```python
from build123d import *

# Parameters (mm, degrees)
SKETCH_1_W          = 60
SKETCH_1_H          = 45
EXTRUDE_1_DEPTH     = 13.5
CHAMFER_1_SIZE      = 10
FILLET_1_R          = 5
SHELL_1_T           = -1.5
FILLET_2_R          = 0.1
SKETCH_4_W          = 42
SKETCH_4_H          = 24
SKETCH_4_W_2        = 38
SKETCH_4_H_2        = 20
EXTRUDE_1_2_DEPTH   = 1
CUT_EXTRUDE_1_REACH = 47.349
SKETCH_7_R          = 2.5


with BuildPart() as part:
    # 草图1 → Extrude 1 (new, symmetric)
    with BuildSketch(Plane(origin=(0, 0, 0), x_dir=(1, 0, 0), z_dir=(0, 1, 0))):
        Rectangle(SKETCH_1_W, SKETCH_1_H)
    extrude(amount=EXTRUDE_1_DEPTH, both=True)

    # 倒角1
    chamfer_1_edges = [part.edges().sort_by_distance(p)[0] for p in [
        (-30, 0, 22.5),
        (-30, 0, -22.5),
    ]]
    chamfer(chamfer_1_edges, length=CHAMFER_1_SIZE)

    # 圆角1
    fillet_1_edges = [part.edges().sort_by_distance(p)[0] for p in [
        (-30, 0, 12.5),
        (-30, 0, -12.5),
        (-20, 0, -22.5),
        (-20, 0, 22.5),
    ]]
    fillet(fillet_1_edges, radius=FILLET_1_R)

    # 抽壳1
    shell_1_openings = [part.faces().sort_by_distance(p)[0] for p in [
        (30, 0, 0),
    ]]
    offset(amount=SHELL_1_T, openings=shell_1_openings, kind=Kind.INTERSECTION)

    # 圆角2
    fillet_2_edges = [part.edges().sort_by_distance(p)[0] for p in [
        (-25, 13.5, -17.5),
        (-30, 13.5, 0),
        (-25, 13.5, 17.5),
        (6.035533906, 13.5, 22.5),
        (-19.84234935, 13.5, 22.119397663),
        (-29.619397663, 13.5, 12.34234935),
        (-29.619397663, 13.5, -12.34234935),
        (-19.84234935, 13.5, -22.119397663),
        (-25, -13.5, -17.5),
        (-30, -13.5, 0),
        (6.035533906, -13.5, 22.5),
        (-25, -13.5, 17.5),
        (-19.84234935, -13.5, 22.119397663),
        (-29.619397663, -13.5, 12.34234935),
        (-29.619397663, -13.5, -12.34234935),
        (-19.84234935, -13.5, -22.119397663),
        (30, 13.5, 0),
        (6.035533906, -13.5, -22.5),
        (30, -12, 0),
        (30, 0, 21),
        (30, 0, -21),
        (30, 12, 0),
        (30, -13.5, 0),
        (6.035533906, 13.5, -22.5),
        (30, 0, 22.5),
        (30, 0, -22.5),
    ]]
    fillet(fillet_2_edges, radius=FILLET_2_R)

    # 草图3 → 旋转1 (revolve)
    with BuildSketch(Plane.XY, mode=Mode.PRIVATE) as revolve_1_sk:
        Polygon((0, 12), (4, 12), (4, 3.5), (14, 3.5), (14, 2.5), (12.5, 2.5), (12.5, -7.5), (14, -7.5), (14, -8.5), (4, -8.5), (4, -12), (0, -12), align=None)
    revolve(revolve_1_sk.sketch.rotate(Axis((0, 13.4, 0), (0, -1, 0)), 90), axis=Axis((0, 13.4, 0), (0, -1, 0)))

    # 草图4 → Extrude 1 2 (add, symmetric)
    with BuildSketch(Plane(origin=(20, 0, 0), x_dir=(0, 0, -1), z_dir=(1, 0, 0))):
        Rectangle(SKETCH_4_W, SKETCH_4_H)
        Rectangle(SKETCH_4_W_2, SKETCH_4_H_2, mode=Mode.SUBTRACT)
    extrude(amount=EXTRUDE_1_2_DEPTH, both=True)

    # 草图7 → 切除-拉伸1 (cut, up to next)
    with BuildSketch(Plane(origin=(0, -12, 0), x_dir=(1, 0, 0), z_dir=(0, 1, 0)), mode=Mode.PRIVATE) as cut_extrude_1_sk1:
        with Locations(Location((25, 0, 0), (0, 0, 270))):
            Circle(SKETCH_7_R)
    cut_extrude_1_tool1 = extrude(cut_extrude_1_sk1.sketch, amount=-CUT_EXTRUDE_1_REACH, mode=Mode.PRIVATE) & part.part
    add(cut_extrude_1_tool1.solids().sort_by_distance((25, -12, 0))[0], mode=Mode.SUBTRACT)


solid = part.part
```
The model under review builds one solid part; all positions refer to its coordinate system, in mm. A direction names the side the tool comes from. Round coordinates to 2 decimals unless told otherwise and drop trailing zeros. Write each loop counter-clockwise with the first axis right and the second up, starting at its lowest first coordinate (ties: lowest second). Pieces come first, ordered by that corner, then holes. Notation, with made-up numbers: (63.25, 21) - (84.25, 21) arc R12 ccw to (84.25, 44) - close; hole circle Ø11 at (-24, 3.5). An arc over 180 degrees is marked (long way). One line per question, with ' | ' between items.
Item 1: Add section D-D, the plane x = -16. Give the boundary of the cut face in (y, z).
Resolved:
outline: (-13.5, -22.4) arc R0.1 ccw to (-13.4, -22.5) - (13.4, -22.5) arc R0.1 ccw to (13.5, -22.4) - (13.5, 22.4) arc R0.1 ccw to (13.4, 22.5) - (-13.4, 22.5) arc R0.1 ccw to (-13.5, 22.4) - close; hole (-12, -21) - (12, -21) - (12, 21) - (-12, 21) - close
Item 2: For P1, Ø10.5, axis at y = -2.5, z = 3, coming from the +X side; P2, Ø7, axis at y = -4, z = -10, coming from the +X side; P3, Ø6, axis at y = -7.5, z = -16.5, coming from the -X side, all flat-tipped, find the tip position at first contact; note any pin that passes through.
Resolved:
P1: stops at x = 13.93 | P2: stops at x = 10.68 | P3: stops at x = -28.95
Item 3: Add section C-C, the plane x = 25. Give the boundary of the cut face in (y, z), then the cut area to 3 significant figures.
Resolved:
outline: (-13.5, -22.4) arc R0.1 ccw to (-13.4, -22.5) - (13.4, -22.5) arc R0.1 ccw to (13.5, -22.4) - (13.5, 22.4) arc R0.1 ccw to (13.4, 22.5) - (-13.4, 22.5) arc R0.1 ccw to (-13.5, 22.4) - (-13.5, 2.5) - (-12, 2.5) - (-12, 21) - (12, 21) - (12, -21) - (-12, -21) - (-12, -2.5) - (-13.5, -2.5) - close | area: 199 mm2
Item 4: For faces 1 (the face through (21, -11, 2)), 2 (the face through (-29.63, 0.19, 12.32)), 3 (the face through (3.905, 7.69, -0.867)), list the 3-axis set-ups (+Z, -Z, +X, -X, +Y, -Y) from which the entire face can be reached by the end or side of a thin tool; tool diameter is ignored.
Resolved:
face 1: +X | face 2: +Z, -X, +Y, -Y | face 3: none
Item 5: The part is to be moulded in two halves that separate along X. For faces 4 (the face through (3, 3.5, -3)), 5 (the face through (-29.63, -0.19, -12.32)), 6 (the face through (0, 13.5, 0)), 7 (the face through (0, 0, -21)), say which applies: pulls with the +X half, pulls with the -X half, needs draft (parallel to the pull), parting line crosses it, or undercut.
Resolved:
face 4: undercut | face 5: pulls with the -X half | face 6: needs draft | face 7: undercut
Item 6: To check wall thickness, follow probe 1 along Y at (x, z) = (9.5, -4); probe 2 along Z at (x, y) = (-18, 1.75); probe 3 along Y at (x, z) = (23.5, -4). State the ranges of each line that lie inside material, in increasing order.
Resolved:
probe 1: y = -13.5 to -12, -8.5 to 3.5, 12 to 13.5 | probe 2: z = -22.5 to -21, 21 to 22.5 | probe 3: y = -13.5 to -12, 12 to 13.5
